Source: CAD feature listing. Evaluate the final solid. Frame: model axes, mm. A direction names the side the tool comes from. Coordinates: 2 decimals unless noted, no trailing zeros. Write each loop counter-clockwise with the first axis right and the second up, starting at its lowest first coordinate (ties: lowest second). Pieces come first, ordered by that corner, then holes. Notation, with made-up numbers: (-40, 31.5) - (-11, 31.5) arc R14 ccw to (-11, 52.5) - close; hole circle Ø2 at (63, 58). An arc over 180 degrees is marked (long way). One line per item, written item: value.
from build123d import *

# Parameters (mm, degrees)
SALIENTE_EXTRUIR1_DEPTH    = 6
REDONDEO1_R                = 8
REDONDEO2_R                = 5
REDONDEO3_R                = 8
REDONDEO4_R                = 0.8
CROQUIS2_R                 = 1.9
CORTAR_EXTRUIR1_DEPTH      = 6
CORTAR_EXTRUIR1_DEPTH_BACK = 6
REDONDEO5_R                = 5
CROQUIS3_R                 = 1.95
CORTAR_EXTRUIR2_DEPTH      = 39.095275313
CORTAR_EXTRUIR2_DEPTH_BACK = 10


with BuildPart() as part:
    # Croquis1 → Saliente-Extruir1 (new body)
    with BuildSketch(Plane(origin=(0, 0, 0), x_dir=(1, 0, 0), z_dir=(0, 1, 0))):
        Polygon((-12, -12), (-9, -12), (3, 0), (0, 0), align=None)
        Polygon((3, 0), (0, 0), (0, 20), (15, 20), (15, 17.5), (3, 17.5), (3, 12.5), (15, 12.5), (15, 10), (3, 10), align=None)
        Polygon((-2, -22), (1, -22), (-9, -12), (-12, -12), align=None)
    extrude(amount=SALIENTE_EXTRUIR1_DEPTH)

    # Redondeo1
    redondeo1_edges = [part.edges().sort_by_distance(p)[0] for p in [
        (-9, 3, 12),
    ]]
    fillet(redondeo1_edges, radius=REDONDEO1_R)

    # Redondeo2
    redondeo2_edges = [part.edges().sort_by_distance(p)[0] for p in [
        (-12, 3, 12),
    ]]
    fillet(redondeo2_edges, radius=REDONDEO2_R)

    # Redondeo3
    redondeo3_edges = [part.edges().sort_by_distance(p)[0] for p in [
        (0, 3, 0),
        (3, 3, 0),
    ]]
    fillet(redondeo3_edges, radius=REDONDEO3_R)

    # Redondeo4
    redondeo4_edges = [part.edges().sort_by_distance(p)[0] for p in [
        (1, 3, 22),
        (-2, 3, 22),
    ]]
    fillet(redondeo4_edges, radius=REDONDEO4_R)

    # Croquis2 → Cortar-Extruir1 (cut, two sides)
    with BuildSketch(Plane(origin=(-10.5, 0, 10.5), x_dir=(-0.7071067811865541, 0, -0.7071067811865409), z_dir=(0.7071067811865409, 0, -0.7071067811865541))) as cortar_extruir1_sk:
        with Locations(Location((-10.332085117, 3, 0), (0, 0, 83.63113879))):
            Circle(CROQUIS2_R)
    extrude(amount=CORTAR_EXTRUIR1_DEPTH, mode=Mode.SUBTRACT)
    extrude(cortar_extruir1_sk.sketch, amount=-CORTAR_EXTRUIR1_DEPTH_BACK, mode=Mode.SUBTRACT)

    # Redondeo5
    redondeo5_edges = [part.edges().sort_by_distance(p)[0] for p in [
        (3, 3, -10),
    ]]
    fillet(redondeo5_edges, radius=REDONDEO5_R)

    # Croquis3 → Cortar-Extruir2 (cut, two sides)
    with BuildSketch(Plane(origin=(0, 0, -12.5), x_dir=(-1, 0, 0), z_dir=(0, 0, -1))) as cortar_extruir2_sk:
        with Locations((-9, 3)):
            Circle(CROQUIS3_R)
    extrude(amount=CORTAR_EXTRUIR2_DEPTH, mode=Mode.SUBTRACT)
    extrude(cortar_extruir2_sk.sketch, amount=-CORTAR_EXTRUIR2_DEPTH_BACK, mode=Mode.SUBTRACT)


solid = part.part
1) Section query A-A on x = 13.25. Output: boundary loops of the cut face in (y, z), then the cut area to 3 significant figures.
Values found:
outline: (0, -20) - (6, -20) - (6, -17.5) - (0, -17.5) - close; (0, -12.5) - (6, -12.5) - (6, -10) - (0, -10) - close
area: 30.0 mm2
2) Section query D-D on z = -13. Output: boundary loops of the cut face in (x, y).
Values found:
outline: (0, 0) - (3, 0) - (3, 6) - (0, 6) - close
3) Reachability of faces 4 (the flat face through (3, 3, -4)), 5 (the flat face through (3, 3, -15)), 6 (the flat face through (-6, 2, 18)) from +Z, -Z, +X, -X, +Y, -Y: full face, straight path, thin tool, end or side. Return the list, or none.
Values found:
face 4: +Z, +X, +Y, -Y
face 5: +X, +Y, -Y
face 6: +Z, -X, +Y, -Y
4) Section query B-B on x = 9. Output: boundary loops of the cut face in (y, z), then the cut area to 3 significant figures.
Values found:
outline: (0, -20) - (1.05, -20) - (1.05, -17.5) - (0, -17.5) - close; (0, -12.5) - (1.05, -12.5) - (1.05, -10) - (0, -10) - close; (4.95, -20) - (6, -20) - (6, -17.5) - (4.95, -17.5) - close; (4.95, -12.5) - (6, -12.5) - (6, -10) - (4.95, -10) - close
area: 10.5 mm2
5) Section query C-C on y = 3. State how many separate pieces and enclosed holes the cut face has, then the cut area to 3 significant figures.
Values found:
separate pieces: 4
enclosed holes: 0
area: 171 mm2
6) Contact query for flat-ended pins moving along their axis: P1, Ø1.8, axis at y = 4.5, z = -12.5, coming from the -X side; P2, Ø3, axis at x = -5.5, y = 4.5, coming from the +Z side; P3, Ø2, axis at x = -2, z = -14.5, coming from the +Y side; P4, Ø1.5, axis at y = 2.5, z = -15, coming from the +X side. Output: stop coordinate, or through.
Values found:
P1: x = 0
P2: z = 19.99
P3: through
P4: x = 3
7) Draft query along Y for faces 1 (the flat face through (-1.5, 3, 19.5)), 2 (the flat face through (2, 6, -2)), 3 (the cylindrical face through (7.14, 3.59, -18.73)). Return one class per face: released by +Y, released by -Y, zero draft, split by the parting line, or undercut.
Values found:
face 1: zero draft
face 2: released by +Y
face 3: undercut
8) Material intervals for line 1 (X direction, y = 3, z = -18.35); line 2 (Y direction, x = 9, z = -10.6); line 3 (Z direction, x = 13, y = 4.75), sorted ascending.
Values found:
line 1: 0 to 7.05, 10.95 to 15
line 2: 0 to 1.05, 4.95 to 6
line 3: -20 to -17.5, -12.5 to -10
